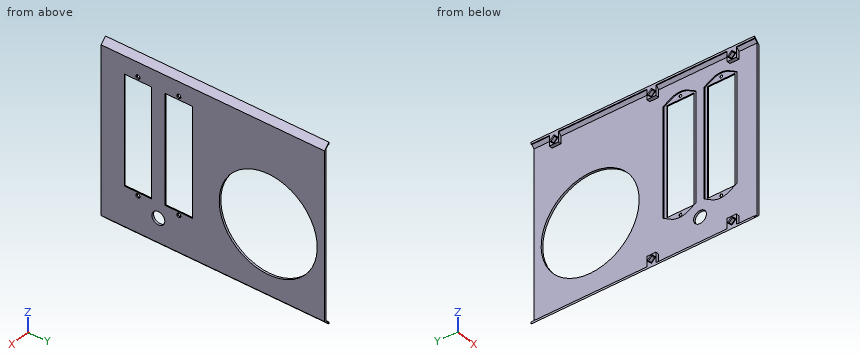
```python
from build123d import *

# Parameters (mm, degrees)
SKETCH1_W                      = 165.076666628
SKETCH1_H                      = 208.28
BOSS_EXTRUDE1_DEPTH            = 5.08
CUT_EXTRUDE1_DEPTH             = 3.175
CUT_EXTRUDE2_REACH             = 134.979
SKETCH8_R                      = 45.72
CUT_EXTRUDE3_REACH             = 134.979
SKETCH9_R                      = 6
SKETCH9_W                      = 101.6
SKETCH9_H                      = 25.4
M2_CLEARANCE_HOLE1_D           = 2.6
M2_CLEARANCE_HOLE1_CSINK_D     = 3.8
M2_CLEARANCE_HOLE1_CSINK_ANGLE = 90
CUT_EXTRUDE4_DEPTH             = 0.9525
CUT_EXTRUDE7_DEPTH             = 4.233333418
CHAMFER1_SIZE                  = 0.635
CHAMFER2_SIZE                  = 2.54
CHAMFER3_SIZE                  = 5.08


with BuildPart() as part:
    # Sketch1 → Boss-Extrude1 (new body)
    with BuildSketch(Plane(origin=(0, 0, 0), x_dir=(0, 0, -1), z_dir=(1, 0, 0))):
        Rectangle(SKETCH1_W, SKETCH1_H)
    extrude(amount=BOSS_EXTRUDE1_DEPTH)

    # Sketch3 → Cut-Extrude1 (cut)
    with BuildSketch(Plane.ZY):
        Polygon((-80.633333314, -12.276666667), (-80.633333314, -78.740000169), (-71.108333314, -78.740000169), (-71.108333314, -87.206666836), (-80.633333314, -87.206666836), (-80.633333314, -104.14), (80.633333314, -104.14), (80.633333314, -87.206666836), (71.108333314, -87.206666836), (71.108333314, -78.740000169), (80.633333314, -78.740000169), (80.633333314, -12.276666667), (71.108333314, -12.276666667), (71.108333314, -3.81), (80.633333314, -3.81), (80.633333314, 78.74), (71.108333314, 78.74), (71.108333314, 87.206666667), (80.633333314, 87.206666667), (80.633333314, 104.14), (-80.633333314, 104.14), (-80.633333314, -3.81), (-71.108333314, -3.81), (-71.108333314, -12.276666667), align=None)
    extrude(amount=-CUT_EXTRUDE1_DEPTH, mode=Mode.SUBTRACT)

    # Sketch8 → Cut-Extrude2 (cut, up to next)
    with BuildSketch(Plane(origin=(5.08, 0, 0), x_dir=(0, 0, -1), z_dir=(1, 0, 0)), mode=Mode.PRIVATE) as cut_extrude2_sk1:
        with Locations((13.288333225, 51.676668489)):
            Circle(SKETCH8_R)
    cut_extrude2_tool1 = extrude(cut_extrude2_sk1.sketch, amount=-CUT_EXTRUDE2_REACH, mode=Mode.PRIVATE) & part.part
    add(cut_extrude2_tool1.solids().sort_by_distance((5.08, 51.676668, -13.288333))[0], mode=Mode.SUBTRACT)

    # Sketch9 → Cut-Extrude3 (cut, up to next)
    with BuildSketch(Plane(origin=(5.08, 0, 0), x_dir=(0, 0, -1), z_dir=(1, 0, 0)), mode=Mode.PRIVATE) as cut_extrude3_sk1:
        with Locations((55.233333314, -50.8)):
            Circle(SKETCH9_R)
    cut_extrude3_tool1 = extrude(cut_extrude3_sk1.sketch, amount=-CUT_EXTRUDE3_REACH, mode=Mode.PRIVATE) & part.part
    # Sketch9 → Cut-Extrude3 (cut, up to next)
    with BuildSketch(Plane(origin=(5.08, 0, 0), x_dir=(0, 0, -1), z_dir=(1, 0, 0)), mode=Mode.PRIVATE) as cut_extrude3_sk2:
        with Locations((-10.148333314, -31.75)):
            Rectangle(SKETCH9_W, SKETCH9_H)
    cut_extrude3_tool2 = extrude(cut_extrude3_sk2.sketch, amount=-CUT_EXTRUDE3_REACH, mode=Mode.PRIVATE) & part.part
    # Sketch9 → Cut-Extrude3 (cut, up to next)
    with BuildSketch(Plane(origin=(5.08, 0, 0), x_dir=(0, 0, -1), z_dir=(1, 0, 0)), mode=Mode.PRIVATE) as cut_extrude3_sk3:
        with Locations((-10.148333314, -69.85)):
            Rectangle(SKETCH9_W, SKETCH9_H)
    cut_extrude3_tool3 = extrude(cut_extrude3_sk3.sketch, amount=-CUT_EXTRUDE3_REACH, mode=Mode.PRIVATE) & part.part
    add(cut_extrude3_tool1.solids().sort_by_distance((5.08, -50.8, -55.233333))[0], mode=Mode.SUBTRACT)
    add(cut_extrude3_tool2.solids().sort_by_distance((5.08, -31.75, 10.148333))[0], mode=Mode.SUBTRACT)
    add(cut_extrude3_tool3.solids().sort_by_distance((5.08, -69.85, 10.148333))[0], mode=Mode.SUBTRACT)

    # M2 Clearance Hole1 (through all)
    with Locations(Plane(origin=(5.08, 0, 0), x_dir=(0, 0, -1), z_dir=(1, 0, 0))):
        with Locations((-64.123333314, -69.85), (43.826666686, -69.85), (43.826666686, -31.75), (-64.123333314, -31.75)):
            CounterSinkHole(M2_CLEARANCE_HOLE1_D / 2, M2_CLEARANCE_HOLE1_CSINK_D / 2, counter_sink_angle=M2_CLEARANCE_HOLE1_CSINK_ANGLE)

    # Sketch12 → Cut-Extrude4 (cut)
    with BuildSketch(Plane.ZY.offset(-3.175)):
        with BuildLine():
            Line((-40.651666686, -16.51), (60.948333314, -16.51))
            Line((60.948333314, -16.51), (65.034587615, -23.682694807))
            ThreePointArc((65.034587615, -23.682694807), (67.171333314, -31.75), (65.034587615, -39.817305193))
            Line((65.034587615, -39.817305193), (60.948333314, -46.99))
            Line((60.948333314, -46.99), (-40.651666686, -46.99))
            Line((-40.651666686, -46.99), (-44.737920986, -39.817305193))
            ThreePointArc((-44.737920986, -39.817305193), (-46.874666686, -31.75), (-44.737920986, -23.682694807))
            Line((-44.737920986, -23.682694807), (-40.651666686, -16.51))
        make_face()
        with BuildLine():
            Line((-44.737920986, -77.917305193), (-40.651666686, -85.09))
            Line((-40.651666686, -85.09), (60.948333314, -85.09))
            Line((60.948333314, -85.09), (65.034587615, -77.917305193))
            ThreePointArc((65.034587615, -77.917305193), (67.171333314, -69.85), (65.034587615, -61.782694807))
            Line((65.034587615, -61.782694807), (60.948333314, -54.61))
            Line((60.948333314, -54.61), (-40.651666686, -54.61))
            Line((-40.651666686, -54.61), (-44.737920986, -61.782694807))
            ThreePointArc((-44.737920986, -61.782694807), (-46.874666686, -69.85), (-44.737920986, -77.917305193))
        make_face()
    extrude(amount=-CUT_EXTRUDE4_DEPTH, mode=Mode.SUBTRACT)

    # Sketch13 → Cut-Extrude7 (cut)
    with BuildSketch(Plane.ZY):
        Polygon((-78.516666732, -8.043333333), (-75.341666732, -4.868333333), (-72.166666732, -8.043333333), (-75.341666732, -11.218333333), align=None)
        Polygon((-78.516666732, -82.973333503), (-75.341666732, -79.798333503), (-72.166666732, -82.973333503), (-75.341666732, -86.148333503), align=None)
        Polygon((72.166666732, -82.973333503), (75.341666732, -79.798333503), (78.516666732, -82.973333503), (75.341666732, -86.148333503), align=None)
        Polygon((72.166666732, -8.043333333), (75.341666732, -4.868333333), (78.516666732, -8.043333333), (75.341666732, -11.218333333), align=None)
        Polygon((72.166666732, 82.973333333), (75.341666732, 86.148333333), (78.516666732, 82.973333333), (75.341666732, 79.798333333), align=None)
    extrude(amount=-CUT_EXTRUDE7_DEPTH, mode=Mode.SUBTRACT)

    # Chamfer1
    chamfer1_edges = [part.edges().sort_by_distance(p)[0] for p in [
        (4.233333418, 81.385833333, 73.754166732),
        (4.233333418, 84.560833333, 73.754166732),
        (4.233333418, 84.560833333, 76.929166732),
        (4.233333418, 81.385833333, 76.929166732),
        (0, 81.385833333, 73.754166732),
        (0, 81.385833333, 76.929166732),
        (0, 84.560833333, 76.929166732),
        (0, 84.560833333, 73.754166732),
        (4.233333418, -9.630833333, 73.754166732),
        (4.233333418, -6.455833333, 73.754166732),
        (4.233333418, -6.455833333, 76.929166732),
        (4.233333418, -9.630833333, 76.929166732),
        (0, -9.630833333, 73.754166732),
        (0, -9.630833333, 76.929166732),
        (0, -6.455833333, 76.929166732),
        (0, -6.455833333, 73.754166732),
        (4.233333418, -84.560833503, 73.754166732),
        (4.233333418, -81.385833503, 73.754166732),
        (4.233333418, -81.385833503, 76.929166732),
        (4.233333418, -84.560833503, 76.929166732),
        (0, -84.560833503, 73.754166732),
        (0, -84.560833503, 76.929166732),
        (0, -81.385833503, 76.929166732),
        (0, -81.385833503, 73.754166732),
        (4.233333418, -84.560833503, -76.929166732),
        (4.233333418, -81.385833503, -76.929166732),
        (4.233333418, -81.385833503, -73.754166732),
        (4.233333418, -84.560833503, -73.754166732),
        (0, -84.560833503, -76.929166732),
        (0, -84.560833503, -73.754166732),
        (0, -81.385833503, -73.754166732),
        (0, -81.385833503, -76.929166732),
        (4.233333418, -9.630833333, -76.929166732),
        (4.233333418, -6.455833333, -76.929166732),
        (4.233333418, -6.455833333, -73.754166732),
        (4.233333418, -9.630833333, -73.754166732),
        (0, -9.630833333, -76.929166732),
        (0, -9.630833333, -73.754166732),
        (0, -6.455833333, -73.754166732),
        (0, -6.455833333, -76.929166732),
    ]]
    chamfer(chamfer1_edges, length=CHAMFER1_SIZE)

    # Chamfer2
    chamfer2_edges = [part.edges().sort_by_distance(p)[0] for p in [
        (3.175, 95.673333333, 80.633333314),
        (3.175, 37.465, 80.633333314),
        (3.175, -45.508333418, 80.633333314),
        (3.175, -95.673333418, 80.633333314),
        (3.175, -95.673333418, -80.633333314),
        (3.175, -45.508333418, -80.633333314),
        (3.175, 50.165, -80.633333314),
    ]]
    chamfer(chamfer2_edges, length=CHAMFER2_SIZE)

    # Chamfer3
    chamfer3_edges = [part.edges().sort_by_distance(p)[0] for p in [
        (5.08, 0, -82.538333314),
        (5.08, 0, 82.538333314),
    ]]
    chamfer(chamfer3_edges, length=CHAMFER3_SIZE - 0.0001)  # a hair under: the kernel refuses the full size


solid = part.part
```
Verification items for the finished model (mm, model axes). Coordinates: 2 decimals unless noted, no trailing zeros. Put each result on its own line as item: value.
Item 1: Scan lines: line 1 along Y through (x, z) = (3.95, 46); line 2 along Z through (x, y) = (4.4, -69.85); line 3 along Z through (x, y) = (4.3, -31.75). Record each from-to range of solid material in increasing order.
Conclusion:
line 1: y = -104.14 to -85.09, -54.61 to -46.99, -16.51 to 104.14
line 2: z = -78.14 to -45.13, -42.53 to -40.65, 60.95 to 62.82, 65.42 to 78.14
line 3: z = -78.24 to -45.13, -42.53 to -40.65, 60.95 to 62.82, 65.42 to 78.24
Item 2: Section check B-B (z = 58). Give the number of separate pieces and of enclosed holes in the cut face, then the cut area to 3 significant figures.
Conclusion:
separate pieces: 3
enclosed holes: 0
area: 290 mm2
Item 3: Gauge pin test, flat ends, axial feed: pin 1 Ø1.6 at (x, z) = (1, 75.5) entering from +Y; pin 2 Ø2.5 at (x, z) = (1.5, 76) entering from -Y; pin 3 Ø2 at (x, y) = (2.5, -79.5) entering from -Z. Record the tip position at first contact, or that the pin passes through.
Conclusion:
pin 1: stops at y = 87.21
pin 2: stops at y = -87.21
pin 3: stops at z = -81.04
